Source: CAD feature listing. Evaluate the final solid. Frame: model axes, mm. A direction names the side the tool comes from. Round coordinates to 2 decimals unless told otherwise and drop trailing zeros. Order: outer loops, then holes, each group sorted by start corner. A loop starts at its lowest first (then second) coordinate and runs counter-clockwise, first axis right, second up. Notation, with made-up numbers: (-35.5, -22) - (11.5, -22) arc R11 ccw to (11.5, -1) - close; hole circle Ø9 at (38, 77). An arc over 180 degrees is marked (long way). Return JSON: item names as keys, results as strings. Group by question number.
1) Section A-A, the plane y = 24.8. Return loops of the section in (x, z).
2) Ray query, line 1 (X direction, y = -3.5, z = 16); line 2 (Y direction, x = -24, z = 22.5); line 3 (X direction, y = -34.5, z = 6.5). Return the intervals inside material, ascending. Write a range as from..to.
3) Access query for faces 5 (the flat face through (-29, 21.371, 24)), 6 (the flat face through (-29, -3, 31.75)), 7 (the flat face through (30, -16, 25.32)), 8 (the cylindrical face through (30.186, -39.705, 22.358)). Directions: +Z, -Z, +X, -X, +Y, -Y. A direction counts if a zero-diameter tool reaches every point of the face in a straight line with its end or side. Return the directions, or none.
4) Contact query for flat-ended pins moving along their axis: P1, Ø3, axis at x = 14.5, y = -5, coming from the +Z side; P2, Ø7.5, axis at x = 23.5, y = 31.5, coming from the +Z side. Output: stop coordinate, or through.
5) Section D-D, the plane x = -9. Return loops of the section in (y, z), plus the area to 4 significant figures.
6) Section B-B, the plane z = 7. Give the number of separate pieces and of enclosed holes in the cut face, plus the area to 3 significant figures.
7) Mould query, pull axis X, two halves, no side actions, for faces 1 (the flat face through (31.21, -41.25, 15.65)), 2 (the flat face through (29, 39, 12.7)), 3 (the flat face through (-30.04, 27.2, 27.5)), 4 (the cylindrical face through (22.97, 35.35, 8.13)). Classes: pulls with the +X half, pulls with the -X half, needs draft (parallel to the pull), parting line crosses it, or undercut.
```python
from build123d import *

# Parameters (mm, degrees)
SKETCH1_W           = 55
SKETCH1_H           = 75
SKETCH1_R           = 0.889
BOSS_EXTRUDE1_DEPTH = 5
SKETCH2_W           = 65
SKETCH2_H           = 85
SKETCH2_W_2         = 55
SKETCH2_H_2         = 75
BOSS_EXTRUDE2_DEPTH = 31.75
CUT_EXTRUDE1_REACH  = 85.901
SKETCH4_R           = 5.207
CUT_EXTRUDE2_DEPTH  = 2.46
CHAMFER1_SIZE       = 2.54
SKETCH5_R           = 0.889
CUT_EXTRUDE3_DEPTH  = 19.05
SKETCH6_R           = 3.429
SKETCH6_R_2         = 0.889
BOSS_EXTRUDE3_DEPTH = 6.35
CUT_EXTRUDE4_REACH  = 85.901
SKETCH7_W           = 13.97
SKETCH7_H           = 17.78
CUT_EXTRUDE5_REACH  = 85.901
SKETCH8_R           = 2.54


with BuildPart() as part:
    # Sketch1 → Boss-Extrude1 (new body)
    with BuildSketch(Plane.XY):
        Rectangle(SKETCH1_W, SKETCH1_H)
        with Locations((-22.225, 32.004)):
            Circle(SKETCH1_R, mode=Mode.SUBTRACT)
        with Locations(Location((-22.225, -32.004, 0), (0, 0, 180))):
            Circle(SKETCH1_R, mode=Mode.SUBTRACT)
        with Locations((22.225, -32.004)):
            Circle(SKETCH1_R, mode=Mode.SUBTRACT)
        with Locations(Location((22.225, 32.004, 0), (0, 0, 180))):
            Circle(SKETCH1_R, mode=Mode.SUBTRACT)
    extrude(amount=BOSS_EXTRUDE1_DEPTH)

    # Sketch2 → Boss-Extrude2 (add)
    with BuildSketch(Plane(origin=(0, 0, 0), x_dir=(-1, 0, 0), z_dir=(0, 0, -1))):
        Rectangle(SKETCH2_W, SKETCH2_H)
        Rectangle(SKETCH2_W_2, SKETCH2_H_2, mode=Mode.SUBTRACT)
    extrude(amount=-BOSS_EXTRUDE2_DEPTH)

    # Sketch3 → Cut-Extrude1 (cut, up to next)
    with BuildSketch(Plane.ZY.offset(32.5), mode=Mode.PRIVATE) as cut_extrude1_sk1:
        with BuildLine():
            Line((25.868155142, 21.371), (22.264844858, 21.371))
            ThreePointArc((22.264844858, 21.371), (20.193, 24.8), (22.264844858, 28.229))
            Line((22.264844858, 28.229), (25.868155142, 28.229))
            ThreePointArc((25.868155142, 28.229), (27.94, 24.8), (25.868155142, 21.371))
        make_face()
    cut_extrude1_tool1 = extrude(cut_extrude1_sk1.sketch, amount=-CUT_EXTRUDE1_REACH, mode=Mode.PRIVATE) & part.part
    add(cut_extrude1_tool1.solids().sort_by_distance((-32.5, 24.8, 24.0665))[0], mode=Mode.SUBTRACT)

    # Sketch4 → Cut-Extrude2 (cut)
    with BuildSketch(Plane.ZY.offset(32.5)):
        with Locations((24.0665, 24.8)):
            Circle(SKETCH4_R)
    extrude(amount=-CUT_EXTRUDE2_DEPTH, mode=Mode.SUBTRACT)

    # Chamfer1
    chamfer1_edges = [part.edges().sort_by_distance(p)[0] for p in [
        (32.5, 42.5, 15.875),
        (-32.5, 42.5, 15.875),
        (-32.5, -42.5, 15.875),
        (32.5, -42.5, 15.875),
    ]]
    chamfer(chamfer1_edges, length=CHAMFER1_SIZE)

    # Sketch5 → Cut-Extrude3 (cut)
    with BuildSketch(Plane.XY.offset(31.75)):
        with Locations((29.365, 39.365)):
            Circle(SKETCH5_R)
        with Locations((29.365, -39.365)):
            Circle(SKETCH5_R)
        with Locations((-29.365, -39.365)):
            Circle(SKETCH5_R)
        with Locations((-29.365, 39.365)):
            Circle(SKETCH5_R)
        with Locations((29.365, 0)):
            Circle(SKETCH5_R)
        with Locations((-29.365, 0)):
            Circle(SKETCH5_R)
    extrude(amount=-CUT_EXTRUDE3_DEPTH, mode=Mode.SUBTRACT)

    # Sketch6 → Boss-Extrude3 (add)
    # profile 1 of 4: a face of its own
    with BuildSketch(Plane.XY.offset(5)):
        with Locations(Location((-22.225, 32.004, 0), (0, 0, 180))):
            Circle(SKETCH6_R)
        with Locations((-22.225, 32.004)):
            Circle(SKETCH6_R_2, mode=Mode.SUBTRACT)
    # profile 2 of 4: a face of its own
    with BuildSketch(Plane.XY.offset(5)):
        with Locations(Location((-22.225, -32.004, 0), (0, 0, 180))):
            Circle(SKETCH6_R)
        with Locations(Location((-22.225, -32.004, 0), (0, 0, 180))):
            Circle(SKETCH6_R_2, mode=Mode.SUBTRACT)
    # profile 3 of 4: a face of its own
    with BuildSketch(Plane.XY.offset(5)):
        with Locations(Location((22.225, -32.004, 0), (0, 0, 180))):
            Circle(SKETCH6_R)
        with Locations((22.225, -32.004)):
            Circle(SKETCH6_R_2, mode=Mode.SUBTRACT)
    # profile 4 of 4: a face of its own
    with BuildSketch(Plane.XY.offset(5)):
        with Locations(Location((22.225, 32.004, 0), (0, 0, 180))):
            Circle(SKETCH6_R)
        with Locations(Location((22.225, 32.004, 0), (0, 0, 180))):
            Circle(SKETCH6_R_2, mode=Mode.SUBTRACT)
    extrude(amount=BOSS_EXTRUDE3_DEPTH)

    # Sketch7 → Cut-Extrude4 (cut, up to next)
    with BuildSketch(Plane(origin=(32.5, 0, 0), x_dir=(0, 0, -1), z_dir=(1, 0, 0)), mode=Mode.PRIVATE) as cut_extrude4_sk1:
        with Locations((-18.335, -15.91)):
            Rectangle(SKETCH7_W, SKETCH7_H)
    cut_extrude4_tool1 = extrude(cut_extrude4_sk1.sketch, amount=-CUT_EXTRUDE4_REACH, mode=Mode.PRIVATE) & part.part
    add(cut_extrude4_tool1.solids().sort_by_distance((32.5, -15.91, 18.335))[0], mode=Mode.SUBTRACT)

    # Sketch8 → Cut-Extrude5 (cut, up to next)
    with BuildSketch(Plane(origin=(32.5, 0, 0), x_dir=(0, 0, -1), z_dir=(1, 0, 0)), mode=Mode.PRIVATE) as cut_extrude5_sk1:
        with Locations((-18.335, -31.15)):
            Circle(SKETCH8_R)
    cut_extrude5_tool1 = extrude(cut_extrude5_sk1.sketch, amount=-CUT_EXTRUDE5_REACH, mode=Mode.PRIVATE) & part.part
    add(cut_extrude5_tool1.solids().sort_by_distance((32.5, -31.15, 18.335))[0], mode=Mode.SUBTRACT)


solid = part.part
```
Geometry check:
{
 "1": {"outline": "(-32.5, 0) - (32.5, 0) - (32.5, 31.75) - (27.5, 31.75) - (27.5, 5) - (-27.5, 5) - (-27.5, 20.19) - (-30.04, 20.19) - (-30.04, 18.86) - (-32.5, 18.86) - close; (-32.5, 29.27) - (-30.04, 29.27) - (-30.04, 27.94) - (-27.5, 27.94) - (-27.5, 31.75) - (-32.5, 31.75) - close"},
 "2": {"line 1": "-32.5..-27.5, 27.5..32.5", "line 2": "-42.5..-37.5, 37.5..42.5", "line 3": "-32.5..-27.5, -24.58..-19.87, 19.87..24.58, 27.5..32.5"},
 "3": {"face 5": "-X", "face 6": "+Z, +X, -X, +Y, -Y", "face 7": "+X", "face 8": "+Z"},
 "4": {"P1": "z = 5", "P2": "z = 11.35"},
 "5": {"outline": "(-42.5, 0) - (42.5, 0) - (42.5, 31.75) - (37.5, 31.75) - (37.5, 5) - (-37.5, 5) - (-37.5, 31.75) - (-42.5, 31.75) - close", "area": "692.5 mm2"},
 "6": {"separate pieces": "5", "enclosed holes": "5", "area": "1,520 mm2"},
 "7": {"face 1": "pulls with the +X half", "face 2": "undercut", "face 3": "pulls with the -X half", "face 4": "undercut"}
}
